Autodesk Inventor part; units mm, degrees
ref_plane "YZ Plane" through (0, 0, 0) normal (1, 0, 0) x (0, 1, 0)
ref_plane "XZ Plane" through (0, 0, 0) normal (0, 1, 0) x (-1, 0, 0)
ref_plane "XY Plane" through (0, 0, 0) normal (0, 0, 1) x (1, 0, 0)
sketch "Sketch1" plane through (0, 0, 0) normal (0, 0, 1) x (1, 0, 0)
  line L0 (-5, 0) -> (5, 0)
  line L1 (5, 0) -> (5, 12)
  line L2 (5, 12) -> (-5, 12)
  line L3 (-5, 12) -> (-5, 0)
  arc A0 (-1.118, 7) -> (1.118, 7) centre (0, 6) ccw
  line L4 (0, 7) -> (-1.118, 7)
  line L5 (-1.118, 7) -> (1.118, 7)
  circle A1 centre (0, 6) radius 1.5
  circle A2 centre (0, 6) radius 1.95
  point P0 (0, 0)
  dimension "d0" = 10
  dimension "d1" = 12
extrude "Extrusion1" add sketch "Sketch1" along normal blind 9.271 contours L4 L5 A0
extrude "Extrusion2" add sketch "Sketch1" along normal blind 0.6 contours A2
extrude "Extrusion3" add sketch "Sketch1" along normal blind 0.6 contours A1 L5 L4
sketch "Sketch2" plane through (0, 6, 0) normal (0, 0, -1) x (-1, 0, 0)
  circle A0 centre (0, 0) radius 1.95
  point P0 (0, -6)
extrude "Extrusion4" add sketch "Sketch1" against normal blind 9 contours L3 L2 L1 L0
extrude "Extrusion5" add sketch "Sketch2" along normal blind 9
sketch "Sketch4" plane through (0, 0, -9) normal (0, 0, -1) x (-1, 0, 0)
  line L0 (5, 9.3166) -> (5, 2.6834)
  line L1 (-5, 2.6834) -> (-5, 9.3166)
  arc A0 (5, 9.3166) -> (-5, 9.3166) centre (0, 6) ccw
  arc A1 (-5, 2.6834) -> (5, 2.6834) centre (0, 6) ccw
  point P0 (0, 0)
extrude "Extrusion6" add sketch "Sketch4" along normal blind 15
sketch "Sketch5" plane through (0, 0, -24) normal (0, 0, -1) x (-1, 0, 0)
  circle A0 centre (0, 6) radius 2.5
  circle A1 centre (0, 6) radius 0.5
  point P0 (0, 0)
extrude "Extrusion7" add sketch "Sketch5" along normal blind 1
extrude "Extrusion8" add sketch "Sketch5" along normal blind 5.5 contours A1
sketch "Sketch6" plane through (-5, 0, 0) normal (0, -1, 0) x (1, 0, 0)
  line L0 (0, 0) -> (10, 0)
  line L1 (0, 0) -> (0, -9)
  line L2 (5, -9) -> (0, -9)
  line L3 (10, -9) -> (5, -9)
  line L4 (10, 0) -> (10, -9)
  line L5 (5, -9) -> (10, -9)
  line L6 (0, -9) -> (5, -9)
  line L7 (0, -9) -> (0, -24)
  line L8 (10, -24) -> (0, -24)
  line L9 (10, -9) -> (10, -24)
  line L10 (0, 0) -> (10, 0)
  line L11 (0, 0) -> (0, -9)
  line L12 (5, -9) -> (0, -9)
  line L13 (10, -9) -> (5, -9)
  line L14 (10, 0) -> (10, -9)
  line L15 (3.882, 0.6) -> (6.118, 0.6)
  line L16 (6.118, 0.6) -> (6.118, 9.271)
  line L17 (3.882, 9.271) -> (6.118, 9.271)
  line L18 (3.882, 0.6) -> (3.882, 9.271)
  line L19 (6.95, 0.6) -> (3.05, 0.6)
  line L20 (3.5, 0.6) -> (3.5, 9.271)
  line L21 (4.5, -29.5) -> (5.5, -29.5)
  line L22 (5.5, -25) -> (4.5, -25)
  line L23 (2.5, -25) -> (7.5, -25)
  line L24 (7.5, -24) -> (2.5, -24)
  line L25 (5.5, -25) -> (5.5, -29.5)
  line L26 (4.5, -25) -> (4.5, -29.5)
  line L27 (2.5, -24) -> (2.5, -25)
  line L28 (2.5, -25) -> (7.5, -25)
  line L29 (7.5, -24) -> (7.5, -25)
  line L30 (6.5, 0.6) -> (6.5, 9.271)
  line L31 (6.95, 0) -> (6.95, 0.6)
  line L32 (3.05, 0) -> (3.05, 0.6)
  line L33 (6.5, 9.271) -> (3.5, 9.271)
  point P0 (5, 0)
properties part number "Motors" material "Stainless Steel"
Input: part model. Units: mm. Frame: model coordinates. A direction names the side the tool comes from. Round coordinates to 2 decimals unless told otherwise and drop trailing zeros. Write each loop counter-clockwise with the first axis right and the second up, starting at its lowest first coordinate (ties: lowest second). Pieces come first, ordered by that corner, then holes. Notation, with made-up numbers: (63, -37.75) - (70, -37.75) arc R25 cw to (70, -6.75) - close; hole circle Ø7 at (-30, 28.5). An arc over 180 degrees is marked (long way). Write item = value, one per line.
(1) Section query C-C on z = -16.5. Output: boundary loops of the cut face in (x, y).
Geometry check:
outline = (-5, 2.68) arc R6 ccw to (5, 2.68) - (5, 9.32) arc R6 ccw to (-5, 9.32) - close
(2) Material intervals for probe 1 along Z at (x, y) = (-3, 4); probe 2 along Z at (x, y) = (-1.5, 7); probe 3 along Y at (x, z) = (0.5, 0.5), sorted ascending.
Geometry check:
probe_1 = -24 to 0
probe_2 = -25 to 0.6
probe_3 = 4.12 to 7.88
(3) Access query for faces 1 (the cylindrical face through (0.33, 3.52, -24.49)), 2 (the cylindrical face through (-1.547, 7.187, 0.296)), 3 (the flat face through (2.2, 11.8, -9)). Directions: +Z, -Z, +X, -X, +Y, -Y. A direction counts if a zero-diameter tool reaches every point of the face in a straight line with its end or side. Return the directions, or none.
Geometry check:
face_1 = -Z
face_2 = +Z
face_3 = -Z, +Y
(4) Section query B-B on y = 6. Output: boundary loops of the cut face in (x, z), then the cut area to 3 significant figures.
Geometry check:
outline = (-5, -24) - (-2.5, -24) - (-2.5, -25) - (-0.5, -25) - (-0.5, -29.5) - (0.5, -29.5) - (0.5, -25) - (2.5, -25) - (2.5, -24) - (5, -24) - (5, 0) - (1.95, 0) - (1.95, 0.6) - (1.5, 0.6) - (1.5, 9.27) - (-1.5, 9.27) - (-1.5, 0.6) - (-1.95, 0.6) - (-1.95, 0) - (-5, 0) - close
area = 278 mm^2
(5) Contact query for flat-ended pins moving along their axis: pin 1 Ø5 at (x, z) = (0.5, 5) entering from -Y; pin 2 Ø4 at (x, y) = (3.5, 7.5) entering from -Z; pin 3 Ø2.5 at (x, z) = (-0.5, 3) entering from +Y. Output: stop coordinate, or through.
Geometry check:
pin_1 = 4.5
pin_2 = -25
pin_3 = 7
